```python
from build123d import *

# Parameters (mm, degrees)
LEG_DEPTH               = 87
SKETCH5_W               = 20
SKETCH5_H               = 21.25
CELL_SLOTS_DEPTH        = 30
SKETCH6_W               = 20
SKETCH6_H               = 0.25
CELL_SLOTS_TRIM_DEPTH   = 30
SKETCH7_R               = 1.8
SCREW_HOLES_FRONT_DEPTH = 10


with BuildPart() as part:
    # Sketch1 → Leg (new, symmetric)
    with BuildSketch(Plane.XY):
        Polygon((0, -6), (0, 0), (0, 30), (-54.5, 30), (-54.5, -6), align=None)
    extrude(amount=LEG_DEPTH, both=True)

    # Sketch5 → Cell Slots (cut)
    with BuildSketch(Plane(origin=(0, 30, 0), x_dir=(1, 0, 0), z_dir=(0, 1, 0))):
        with Locations((-10, -81.375)):
            Rectangle(SKETCH5_W, SKETCH5_H)
        with Locations((-10, -58.125)):
            Rectangle(SKETCH5_W, SKETCH5_H)
        with Locations((-10, -34.875)):
            Rectangle(SKETCH5_W, SKETCH5_H)
        with Locations((-10, -11.625)):
            Rectangle(SKETCH5_W, SKETCH5_H)
        with Locations((-10, 11.625)):
            Rectangle(SKETCH5_W, SKETCH5_H)
        with Locations((-10, 34.875)):
            Rectangle(SKETCH5_W, SKETCH5_H)
        with Locations((-10, 58.125)):
            Rectangle(SKETCH5_W, SKETCH5_H)
        with Locations((-10, 81.375)):
            Rectangle(SKETCH5_W, SKETCH5_H)
        with Locations((-44.5, -81.375)):
            Rectangle(SKETCH5_W, SKETCH5_H)
        with Locations((-44.5, -58.125)):
            Rectangle(SKETCH5_W, SKETCH5_H)
        with Locations((-44.5, -34.875)):
            Rectangle(SKETCH5_W, SKETCH5_H)
        with Locations((-44.5, -11.625)):
            Rectangle(SKETCH5_W, SKETCH5_H)
        with Locations((-44.5, 11.625)):
            Rectangle(SKETCH5_W, SKETCH5_H)
        with Locations((-44.5, 34.875)):
            Rectangle(SKETCH5_W, SKETCH5_H)
        with Locations((-44.5, 58.125)):
            Rectangle(SKETCH5_W, SKETCH5_H)
        with Locations((-44.5, 81.375)):
            Rectangle(SKETCH5_W, SKETCH5_H)
    extrude(amount=-CELL_SLOTS_DEPTH, mode=Mode.SUBTRACT)

    # Sketch6 → Cell Slots Trim (cut)
    with BuildSketch(Plane(origin=(0, 30, 0), x_dir=(1, 0, 0), z_dir=(0, 1, 0))):
        with Locations((-10, -70.625)):
            Rectangle(SKETCH6_W, SKETCH6_H)
        with Locations((-10, -68.875)):
            Rectangle(SKETCH6_W, SKETCH6_H)
        with Locations((-10, -47.375)):
            Rectangle(SKETCH6_W, SKETCH6_H)
        with Locations((-10, -45.625)):
            Rectangle(SKETCH6_W, SKETCH6_H)
        with Locations((-10, -24.125)):
            Rectangle(SKETCH6_W, SKETCH6_H)
        with Locations((-10, -22.375)):
            Rectangle(SKETCH6_W, SKETCH6_H)
        with Locations((-10, -0.875)):
            Rectangle(SKETCH6_W, SKETCH6_H)
        with Locations((-10, 0.875)):
            Rectangle(SKETCH6_W, SKETCH6_H)
        with Locations((-10, 22.375)):
            Rectangle(SKETCH6_W, SKETCH6_H)
        with Locations((-10, 24.125)):
            Rectangle(SKETCH6_W, SKETCH6_H)
        with Locations((-10, 45.625)):
            Rectangle(SKETCH6_W, SKETCH6_H)
        with Locations((-10, 47.375)):
            Rectangle(SKETCH6_W, SKETCH6_H)
        with Locations((-10, 68.875)):
            Rectangle(SKETCH6_W, SKETCH6_H)
        with Locations((-10, 70.625)):
            Rectangle(SKETCH6_W, SKETCH6_H)
        with Locations((-44.5, 70.625)):
            Rectangle(SKETCH6_W, SKETCH6_H)
        with Locations((-44.5, 68.875)):
            Rectangle(SKETCH6_W, SKETCH6_H)
        with Locations((-44.5, 47.375)):
            Rectangle(SKETCH6_W, SKETCH6_H)
        with Locations((-44.5, 45.625)):
            Rectangle(SKETCH6_W, SKETCH6_H)
        with Locations((-44.5, 24.125)):
            Rectangle(SKETCH6_W, SKETCH6_H)
        with Locations((-44.5, 22.375)):
            Rectangle(SKETCH6_W, SKETCH6_H)
        with Locations((-44.5, 0.875)):
            Rectangle(SKETCH6_W, SKETCH6_H)
        with Locations((-44.5, -0.875)):
            Rectangle(SKETCH6_W, SKETCH6_H)
        with Locations((-44.5, -22.375)):
            Rectangle(SKETCH6_W, SKETCH6_H)
        with Locations((-44.5, -24.125)):
            Rectangle(SKETCH6_W, SKETCH6_H)
        with Locations((-44.5, -45.625)):
            Rectangle(SKETCH6_W, SKETCH6_H)
        with Locations((-44.5, -47.375)):
            Rectangle(SKETCH6_W, SKETCH6_H)
        with Locations((-44.5, -68.875)):
            Rectangle(SKETCH6_W, SKETCH6_H)
        with Locations((-44.5, -70.625)):
            Rectangle(SKETCH6_W, SKETCH6_H)
    extrude(amount=-CELL_SLOTS_TRIM_DEPTH, mode=Mode.SUBTRACT)

    # Sketch7 → Screw Holes Front (cut)
    with BuildSketch(Plane.XY.offset(87)):
        with Locations((-33.25, -3)):
            Circle(SKETCH7_R)
        with Locations(Location((-21.25, -3, 0), (0, 0, 180))):
            Circle(SKETCH7_R)
    screw_holes_front = extrude(amount=-SCREW_HOLES_FRONT_DEPTH, mode=Mode.SUBTRACT)

    # Screw Holes Back: Screw Holes Front across plane
    add(screw_holes_front.mirror(Plane(origin=(0, 0, 0), x_dir=(1, 0, 0), z_dir=(0, 0, -1))), mode=Mode.SUBTRACT)


solid = part.part
```
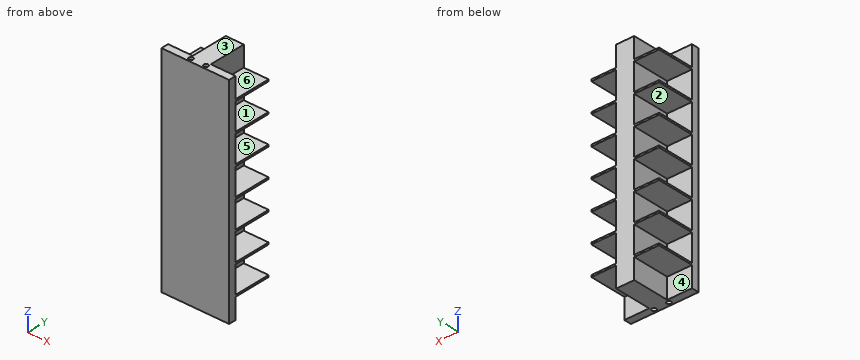
Read the model definition and answer for the solid it produces. Units are mm, in the model's axes. Face numbers are marked on the shaded views. A direction names the side the tool comes from. Coordinates: 2 decimals unless noted, no trailing zeros. Write each loop counter-clockwise with the first axis right and the second up, starting at its lowest first coordinate (ties: lowest second). Pieces come first, ordered by that corner, then holes. Notation, with made-up numbers: (-32.75, 50.25) -> (19.25, 50.25) arc R32 ccw to (19.25, 79.25) -> close; hole circle Ø2 at (41, 60). An arc over 180 degrees is marked (long way). Return JSON: item names as keys, results as strings.
1. Each of these flat-tipped pins is pushed along its axis until it touches: P1, Ø2, axis at y = 9, z = -37.5, coming from the -X side; P2, Ø6, axis at x = -42.5, y = 10, coming from the +Z side; P3, Ø4, axis at y = 7.5, z = -35.5, coming from the +X side. Where does it stop, or does it pass through?
Found:
{"P1": "x = -34.5", "P2": "z = 70.5", "P3": "x = -20"}
2. A tool of negligible diameter and unlimited length cuts with its end or side. For the marked faces 1, 2 and 3, from which of +Z, -Z, +X, -X, +Y, -Y can it reach the whole face along a straight path? Write none if from no direction.
Found:
{"face 1": "+X, +Y", "face 2": "-X, +Y", "face 3": "+Z, +X, -X, +Y, -Y"}
3. A cutting plane is placed at B-B (z = 34.5). Determine the outline of the cut face in (x, y).
Found:
{"outline": "(-54.5, -6) -> (0, -6) -> (0, 0) -> (-20, 0) -> (-20, 30) -> (-34.5, 30) -> (-34.5, 0) -> (-54.5, 0) -> close"}
4. Find the intervals of material crossed by line 1 along Y through (x, z) = (-21.25, 82.25); line 2 along Y through (x, z) = (-44.5, 59); line 3 along Y through (x, z) = (-34, -80), in increasing order. Write a range as from..to.
Found:
{"line 1": "-6..-4.8, -1.2..30", "line 2": "-6..0", "line 3": "-6..-4.64, -1.36..30"}
5. A cutting plane is placed at A-A (y = -3). Determine the outline of the cut face in (x, z).
Found:
{"outline": "(-54.5, -87) -> (-35.05, -87) -> (-35.05, -77) -> (-31.45, -77) -> (-31.45, -87) -> (-23.05, -87) -> (-23.05, -77) -> (-19.45, -77) -> (-19.45, -87) -> (0, -87) -> (0, 87) -> (-19.45, 87) -> (-19.45, 77) -> (-23.05, 77) -> (-23.05, 87) -> (-31.45, 87) -> (-31.45, 77) -> (-35.05, 77) -> (-35.05, 87) -> (-54.5, 87) -> close"}
6. Determine the mould class of the marked faces 4, 5 and 6 for opening direction Z: pulls with the +Z half, pulls with the -Z half, needs draft (parallel to the pull), parting line crosses it, or undercut.
Found:
{"face 4": "needs draft", "face 5": "undercut", "face 6": "pulls with the +Z half"}
